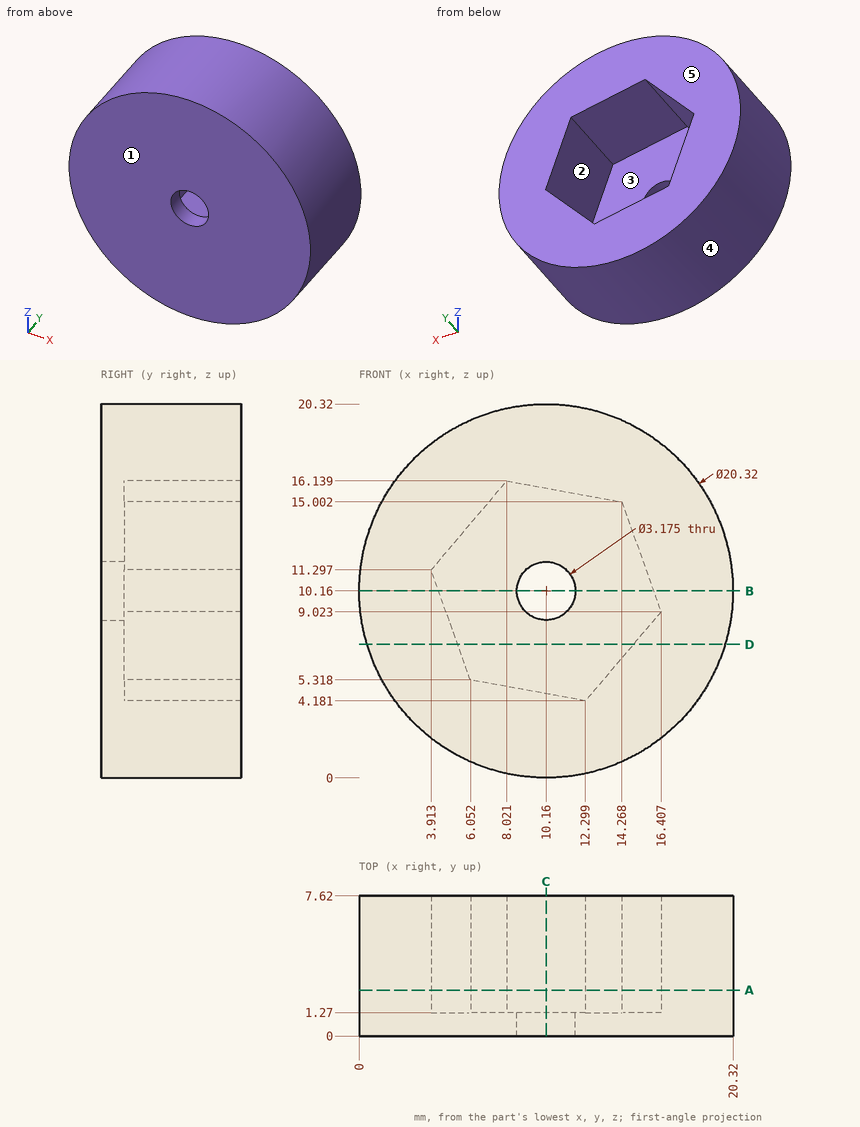
Study the drawing (mm; zero at the part's minimum x, y, z) and answer. A direction names the side the tool comes from. Give positions to 0.01 mm unless a question says otherwise; leave off trailing zeros. Write each loop counter-clockwise with the first axis right and the second up, starting at its lowest first coordinate (ties: lowest second). Pieces come first, ordered by that corner, then holes. Notation, with made-up numbers: (36, 1.25) -> (76, 1.25) arc R12 cw to (76, 7.25) -> close; hole circle Ø5 at (65.5, 70.5). An arc over 180 degrees is marked (long way). Answer in a Markdown table with one row per item.
1) Determine the mould class of the marked faces 3, 4 and 5 for opening direction X: released by +X, released by -X, zero draft, split by the parting line, or undercut.
Results list:
| item | result |
|---|---|
| face 3 | undercut |
| face 4 | split by the parting line |
| face 5 | zero draft |
2) A tool of negligible diameter and unlimited length cuts with its end or side. For the marked faces 1 and 2, from which of +Z, -Z, +X, -X, +Y, -Y can it reach the whole face along a straight path? Write none if from no direction.
Results list:
| item | result |
|---|---|
| face 1 | +Z, -Z, +X, -X, -Y |
| face 2 | +Y |
3) Straight lines are drawn through the part: line 1 (X direction, y = 0.75, z = 10.16); line 2 (X direction, y = 4, z = 6.25) (1 decimal); line 3 (Y direction, x = 13.75, z = 8). For each, find the intervals that lie inside material, in ascending order. Write a range as [from, to].
Results list:
| item | result |
|---|---|
| line 1 | [0, 8.57], [11.75, 20.32] |
| line 2 | [0.8, 5.7], [14.1, 19.5] |
| line 3 | [0, 1.27] |
4) Section D-D on z = 7.25 is taken. Give the vertices of the cut face in (x, y) (1 decimal).
Results list:
| item | result |
|---|---|
| outline | (0.4, 0) -> (19.9, 0) -> (19.9, 7.6) -> (14.9, 7.6) -> (14.9, 1.3) -> (5.4, 1.3) -> (5.4, 7.6) -> (0.4, 7.6) -> close |
5) Section B-B on z = 10.16 is taken. Give the vertices of the cut face in (x, y).
Results list:
| item | result |
|---|---|
| outline | (0, 0) -> (8.57, 0) -> (8.57, 1.27) -> (4.32, 1.27) -> (4.32, 7.62) -> (0, 7.62) -> close; (11.75, 0) -> (20.32, 0) -> (20.32, 7.62) -> (16, 7.62) -> (16, 1.27) -> (11.75, 1.27) -> close |
6) Each of these flat-tipped pins is pushed along its axis until it touches: pin 1 Ø4 at (x, y) = (13, 2) entering from +Z (1 decimal); pin 2 Ø5 at (x, z) = (10.16, 10.16) entering from +Y; pin 3 Ø3 at (y, z) = (3.5, 17) entering from +X. Where does it stop, or does it pass through?
Results list:
| item | result |
|---|---|
| pin 1 | z = 20.3 |
| pin 2 | y = 1.27 |
| pin 3 | x = 18.8 |
7) Section A-A on y = 2.5 is taken. Give the vertices of the cut face in (x, z).
Results list:
| item | result |
|---|---|
| outline | circle Ø20.32 at (10.16, 10.16); hole (3.91, 11.3) -> (6.05, 5.32) -> (12.3, 4.18) -> (16.41, 9.02) -> (14.27, 15) -> (8.02, 16.14) -> close |
8) Section C-C on x = 10.16 is taken. Give the vertices of the cut face in (y, z).
Results list:
| item | result |
|---|---|
| outline | (0, 0) -> (7.62, 0) -> (7.62, 4.57) -> (1.27, 4.57) -> (1.27, 8.57) -> (0, 8.57) -> close; (0, 11.75) -> (1.27, 11.75) -> (1.27, 15.75) -> (7.62, 15.75) -> (7.62, 20.32) -> (0, 20.32) -> close |
